For this review, take the finished solid that the model builds, in its own axes (mm). Round coordinates to 2 decimals unless told otherwise and drop trailing zeros. Order: outer loops, then holes, each group sorted by start corner. A loop starts at its lowest first (then second) coordinate and runs counter-clockwise, first axis right, second up. Notation, with made-up numbers: (33.25, 84.5) -> (40.25, 84.5) arc R28 cw to (40.25, 104.5) -> close; hole circle Ø9 at (-31.5, 78). An arc over 180 degrees is marked (long way). Answer in a Markdown table with one row per item.
```python
from build123d import *

# Parameters (mm, degrees)
SKETCH1_W           = 152.4
SKETCH1_H           = 19.05
BOSS_EXTRUDE1_DEPTH = 36.6776
SKETCH2_R           = 4.7625
CUT_EXTRUDE1_DEPTH  = 19.05


with BuildPart() as part:
    # Sketch1 → Boss-Extrude1 (new body, symmetric)
    with BuildSketch(Plane(origin=(0, 0, 0), x_dir=(1, 0, 0), z_dir=(0, 1, 0))):
        Rectangle(SKETCH1_W, SKETCH1_H)
    extrude(amount=BOSS_EXTRUDE1_DEPTH, both=True)

    # Sketch2 → Cut-Extrude1 (cut)
    with BuildSketch(Plane(origin=(0, 36.6776, 0), x_dir=(1, 0, 0), z_dir=(0, 1, 0))):
        with Locations((-57.15, 0)):
            Circle(SKETCH2_R)
        with Locations((57.15, 0)):
            Circle(SKETCH2_R)
    cut_extrude1 = extrude(amount=-CUT_EXTRUDE1_DEPTH, mode=Mode.SUBTRACT)

    # Mirror2: Cut-Extrude1 across plane
    add(cut_extrude1.mirror(Plane.ZX), mode=Mode.SUBTRACT)


solid = part.part
```
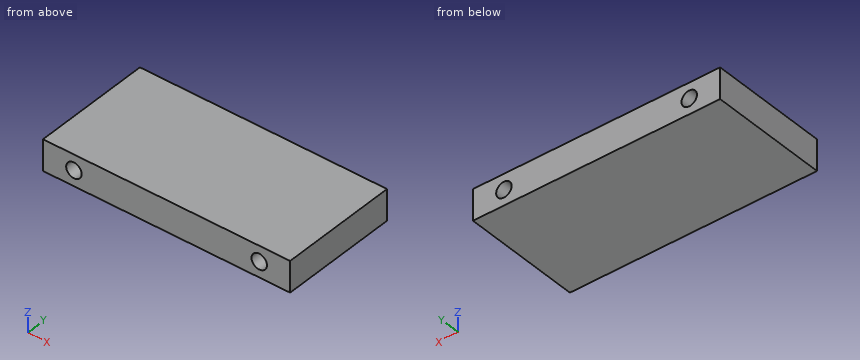
Q1. Take a section at C-C, the plane x = -57.15. Write out the cut boundary in (y, z) (1 decimal).
Answer key:
| item | result |
|---|---|
| outline | (-36.7, -9.5) -> (36.7, -9.5) -> (36.7, -4.8) -> (17.6, -4.8) -> (17.6, 4.8) -> (36.7, 4.8) -> (36.7, 9.5) -> (-36.7, 9.5) -> (-36.7, 4.8) -> (-17.6, 4.8) -> (-17.6, -4.8) -> (-36.7, -4.8) -> close |
Q2. Clearance check with flat-ended pins moving along their axes: pin 1 Ø10.5 at (x, z) = (55, -0.5) entering from -Y; pin 2 Ø3 at (x, z) = (58.5, -0.5) entering from +Y. State where each tip first meets the part, or that it passes through.
Answer key:
| item | result |
|---|---|
| pin 1 | stops at y = -36.68 |
| pin 2 | stops at y = 17.63 |
Q3. Take a section at B-B, the plane y = 30.5. Give the number of separate pieces and of enclosed holes in the cut face, then the cut area to 3 significant figures.
Answer key:
| item | result |
|---|---|
| separate pieces | 1 |
| enclosed holes | 2 |
| area | 2,760 mm^2 |
Q4. To check wall thickness, follow probe 1 along X at (y, z) = (24, 0); probe 2 along Z at (x, y) = (-57, 23) (3 decimals); probe 3 along X at (y, z) = (29.5, -1.25). State the ranges of each line that lie inside material, in increasing order.
Answer key:
| item | result |
|---|---|
| probe 1 | x = -76.2 to -61.91, -52.39 to 52.39, 61.91 to 76.2 |
| probe 2 | z = -9.525 to -4.76, 4.76 to 9.525 |
| probe 3 | x = -76.2 to -61.75, -52.55 to 52.55, 61.75 to 76.2 |
Q5. Take a section at A-A, the plane z = 0. Write out the cut boundary in (x, y), then the cut area to 3 significant figures.
Answer key:
| item | result |
|---|---|
| outline | (-76.2, -36.68) -> (-61.91, -36.68) -> (-61.91, -17.63) -> (-52.39, -17.63) -> (-52.39, -36.68) -> (52.39, -36.68) -> (52.39, -17.63) -> (61.91, -17.63) -> (61.91, -36.68) -> (76.2, -36.68) -> (76.2, 36.68) -> (61.91, 36.68) -> (61.91, 17.63) -> (52.39, 17.63) -> (52.39, 36.68) -> (-52.39, 36.68) -> (-52.39, 17.63) -> (-61.91, 17.63) -> (-61.91, 36.68) -> (-76.2, 36.68) -> close |
| area | 10,500 mm^2 |
